Source: CAD feature listing. Evaluate the final solid. Frame: model axes, mm. Face numbers are marked on the shaded views. A direction names the side the tool comes from. Give positions to 0.01 mm unless a question says otherwise; leave off trailing zeros. Order: outer loops, then holes, each group sorted by start corner. A loop starts at its lowest first (then second) coordinate and runs counter-clockwise, first axis right, second up.
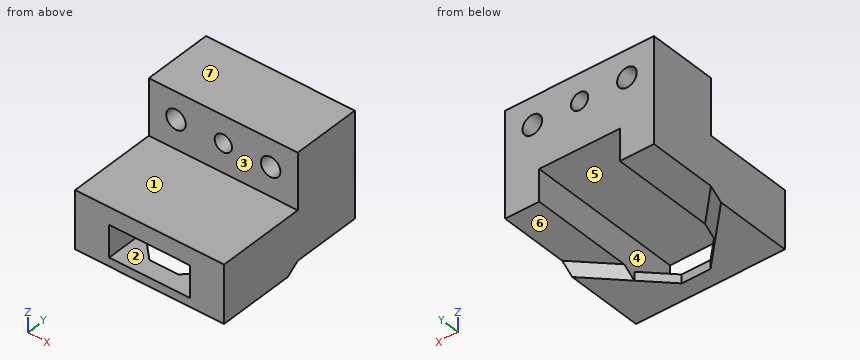
from build123d import *

# Parameters (mm, degrees)
SKETCH1_R           = 1.7
SKETCH1_R_2         = 1.5
BOSS_EXTRUDE1_DEPTH = 12
BOSS_EXTRUDE2_DEPTH = 15.5
SKETCH5_W           = 25.8
SKETCH5_H           = 1.5
BOSS_EXTRUDE3_DEPTH = 3
BOSS_EXTRUDE4_DEPTH = 1.5
CHAMFER1_SIZE       = 1.5


with BuildPart() as part:
    # Sketch1 → Boss-Extrude1 (new body)
    with BuildSketch(Plane(origin=(0, 0, 0), x_dir=(1, 0, 0), z_dir=(0, 1, 0))):
        Polygon((0, 0), (25.8, 0), (25.8, 18.2), (19.9, 18.2), (19.9, 12.7), (5.9, 12.7), (5.9, 18.2), (0, 18.2), align=None)
        with Locations(Location((4.7, 4.7, 0), (0, 0, 270))):
            Circle(SKETCH1_R, mode=Mode.SUBTRACT)
        with Locations(Location((12.9, 4.7, 0), (0, 0, 270))):
            Circle(SKETCH1_R_2, mode=Mode.SUBTRACT)
        with Locations(Location((21.1, 4.7, 0), (0, 0, 270))):
            Circle(SKETCH1_R, mode=Mode.SUBTRACT)
    extrude(amount=BOSS_EXTRUDE1_DEPTH)

    # Sketch4 → Boss-Extrude2 (add)
    with BuildSketch(Plane.XZ):
        Polygon((19.9, -18.2), (19.9, -12.7), (5.9, -12.7), (5.9, -18.2), (0, -18.2), (0, -9.7), (25.8, -9.7), (25.8, -18.2), align=None)
    extrude(amount=BOSS_EXTRUDE2_DEPTH)

    # Sketch5 → Boss-Extrude3 (add)
    with BuildSketch(Plane.XZ.offset(15.5)):
        with Locations((12.9, -18.95)):
            Rectangle(SKETCH5_W, SKETCH5_H)
    extrude(amount=-BOSS_EXTRUDE3_DEPTH)

    # Sketch6 → Boss-Extrude4 (add)
    with BuildSketch(Plane(origin=(0, 0, -19.7), x_dir=(-1, 0, 0), z_dir=(0, 0, -1))):
        Polygon((-25.8, -12.5), (-25.8, -2.1), (-15.4, -12.5), align=None)
        Polygon((0, -12.5), (-10.4, -12.5), (0, -2.1), align=None)
    extrude(amount=-BOSS_EXTRUDE4_DEPTH)

    # Chamfer1
    chamfer1_edges = [part.edges().sort_by_distance(p)[0] for p in [
        (22.85, -5.05, -18.2),
        (2.95, -5.05, -18.2),
    ]]
    chamfer(chamfer1_edges, length=CHAMFER1_SIZE - 0.0001)  # a hair under: the kernel refuses the full size


solid = part.part
1) Section query B-B on y = 1.5. Output: boundary loops of the cut face in (x, z), and give its area (3 significant figures).
Checks:
outline: (0, -18.2) - (5.9, -18.2) - (5.9, -12.7) - (19.9, -12.7) - (19.9, -18.2) - (25.8, -18.2) - (25.8, 0) - (0, 0) - close; hole circle Ø3.4 at (4.7, -4.7); hole circle Ø3 at (12.9, -4.7); hole circle Ø3.4 at (21.1, -4.7)
area: 367 mm2
2) Ray query, L1, parallel to X at y = 6.75, z = -4.7; L2, parallel to X at y = 6, z = -14.75; L3, parallel to Y at x = 21.75, z = -8.5. Return the intervals inside material, ascending.
Checks:
L1: x = 0 to 3, 6.4 to 11.4, 14.4 to 19.4, 22.8 to 25.8
L2: x = 0 to 5.9, 19.9 to 25.8
L3: y = 0 to 12
3) Pull-direction query (Z, two-part tool) for the marked faces 1, 2, 3 and 4; classes: +Z half, -Z half, draft (parallel to the pull), parting line (faces both ways), or undercut.
Checks:
face 1: +Z half
face 2: undercut
face 3: draft
face 4: undercut
4) Reachability of the marked faces 5, 6 and 7 from +Z, -Z, +X, -X, +Y, -Y: full face, straight path, thin tool, end or side. Return the list, or none.
Checks:
face 5: +Y, -Y
face 6: -Z, +Y
face 7: +Z, +X, -X, +Y, -Y
5) Section query D-D on x = 9.75. Output: boundary loops of the cut face in (y, z).
Checks:
outline: (-15.5, -19.7) - (-11.85, -19.7) - (-11.85, -18.2) - (-15.5, -18.2) - close; (-15.5, -12.7) - (12, -12.7) - (12, 0) - (0, 0) - (0, -9.7) - (-15.5, -9.7) - close
6) Section query A-A on z = -17.75. Output: boundary loops of the cut face in (x, y).
Checks:
outline: (0, -15.5) - (5.9, -15.5) - (5.9, 12) - (0, 12) - close; (19.9, -15.5) - (25.8, -15.5) - (25.8, 12) - (19.9, 12) - close
7) Section query C-C on x = 12.9. Output: boundary loops of the cut face in (y, z), and give its area (3 significant figures).
Checks:
outline: (-15.5, -19.7) - (-12.5, -19.7) - (-12.5, -18.2) - (-15.5, -18.2) - close; (-15.5, -12.7) - (12, -12.7) - (12, -6.2) - (0, -6.2) - (0, -9.7) - (-15.5, -9.7) - close; (0, -3.2) - (12, -3.2) - (12, 0) - (0, 0) - close
area: 167 mm2
8) First-contact query: pin 1 Ø3 at (x, y) = (2.5, -1.5) entering from -Z; pin 2 Ø4 at (x, z) = (21.1, -4.7) entering from -Y; pin 3 Ø1.2 at (x, z) = (12.5, -19) entering from +Y. Flat tips, straight axial feed; report the tip coordinate or a pass-through.
Checks:
pin 1: stops at z = -19.01
pin 2: stops at y = 0
pin 3: stops at y = -12.5
